For this review, take the finished solid that the model builds, in its own axes (mm). A direction names the side the tool comes from. Coordinates: 2 decimals unless noted, no trailing zeros. Loops run counter-clockwise (first coordinate to the right, second up) from the corner with the lowest first, then second, coordinate; pieces in that order, holes last. Notation, with made-up numbers: (-35, 19.25) - (15, 19.25) arc R30 ccw to (15, 57.25) - close; hole circle Ø3 at (60.25, 55). An arc over 180 degrees is marked (long way). Answer as a JSON object with one key per item and string values. Group by question number.
Item 1: Clearance check with flat-ended pins moving along their axes: pin 1 (12 mm diameter, centred on y = -629, z = 201, fed in from -X); pin 2 (12 mm diameter, centred on x = -1026, z = 425, fed in from +Y); pin 3 (3 mm diameter, centred on y = -53.5, z = 807.5, fed in from -X). State where each tip first meets the part, or that it passes through.
Item 2: Mouldability with a two-part tool opening along Z and no side actions: class faces 4 (the flat face through (-1026, -628, 810)), 5 (the flat face through (-1048, -628, 800)), 6 (the flat face through (-746, -609.913, 20)) as released by +Z, released by -Z, zero draft, split by the parting line, or undercut.
Item 3: We need section A-A (x = -589.5). Give the boundary of the cut face in (y, z), then the cut area to 3 significant figures.
Item 4: We need section D-D (x = -1019.5). Give the boundary of the cut face in (y, z), then the cut area to 3 significant figures.
Item 5: We need section C-C (y = -482). Give the boundary of the cut face in (x, z), then the cut area to 3 significant figures.
Item 6: We need section B-B (z = 541). Give the boundary of the cut face in (x, y).
Item 7: To check wall thickness, follow line 1 (X direction, y = -628, z = 774.5); line 2 (Y direction, x = -1016.5, z = 723.5); line 3 (Z direction, x = -1004.5, y = -212). State the ranges of each line that lie inside material, in increasing order.
Item 8: Tool access review of faces 1 (the flat face through (-1042.783, -630, 394)), 2 (the flat face through (-1002.783, -630, 415)), 3 (the flat face through (-1022, -49, 800)): name each direction out of +Z, -Z, +X, -X, +Y, -Y from which nothing blocks a thin tool from reaching the whole face with its end or side.
from build123d import *

# Parameters (mm, degrees)
F0_W     = 600
F0_H     = 600
F0_W_2   = 520
F0_H_2   = 520
F1_DEPTH = 40
F2_W     = 40
F2_H     = 40
F3_DEPTH = 800
F4_W     = 100
F4_H     = 100
F4_R     = 5
F5_DEPTH = 10


with BuildPart() as f1:
    # F0 (on Top) → F1 (new body)
    with BuildSketch(Plane.XY):
        with Locations((-742.534351, -349.912536)):
            Rectangle(F0_W, F0_H)
        with Locations((-742.534351, -349.912536)):
            Rectangle(F0_W_2, F0_H_2, mode=Mode.SUBTRACT)
    extrude(amount=F1_DEPTH)

    # F2 (on Top) → F3 (join)
    with BuildSketch(Plane.XY):
        with Locations((-462.971604, -70.520664)):
            Rectangle(F2_W, F2_H)
        with Locations((-1021.841088, -70.520664)):
            Rectangle(F2_W, F2_H)
        with Locations((-462.971604, -629.829387)):
            Rectangle(F2_W, F2_H)
        with Locations((-1022.782568, -629.829387)):
            Rectangle(F2_W, F2_H)
    extrude(amount=F3_DEPTH)

    # F4 (on face) → F5 (join)
    with BuildSketch(Plane.XY.offset(800)):
        with Locations((-1021.178722, -71.567007)):
            Rectangle(F4_W, F4_H)
        with Locations((-1055.047035, -105.544642)):
            Circle(F4_R, mode=Mode.SUBTRACT)
        with Locations((-985.77106, -105.544642)):
            Circle(F4_R, mode=Mode.SUBTRACT)
        with BuildLine():
            ThreePointArc((-1059.987431, -35.498975), (-1055.433054, -29.744166), (-1050.047035, -34.729242))
            ThreePointArc((-1050.047035, -34.729242), (-1050.061959, -35.115261), (-1050.106639, -35.498975))
            ThreePointArc((-1050.106639, -35.498975), (-1050.061959, -35.882689), (-1050.047035, -36.268707))
            ThreePointArc((-1050.047035, -36.268707), (-1055.433054, -41.253784), (-1059.987431, -35.498975))
        make_face(mode=Mode.SUBTRACT)
        with Locations((-985.77106, -36.268707)):
            Circle(F4_R, mode=Mode.SUBTRACT)
        with Locations((-465.089649, -71.444585)):
            Rectangle(F4_W, F4_H)
        with Locations((-498.957962, -105.42222)):
            Circle(F4_R, mode=Mode.SUBTRACT)
        with Locations((-429.681987, -105.42222)):
            Circle(F4_R, mode=Mode.SUBTRACT)
        with BuildLine():
            ThreePointArc((-503.898358, -35.376553), (-499.34398, -29.621744), (-493.957962, -34.606821))
            ThreePointArc((-493.957962, -34.606821), (-493.972885, -34.992839), (-494.017566, -35.376553))
            ThreePointArc((-494.017566, -35.376553), (-493.972885, -35.760268), (-493.957962, -36.146286))
            ThreePointArc((-493.957962, -36.146286), (-499.34398, -41.131363), (-503.898358, -35.376553))
        make_face(mode=Mode.SUBTRACT)
        with Locations((-429.681987, -36.146286)):
            Circle(F4_R, mode=Mode.SUBTRACT)
        with Locations((-463.392437, -630.738995)):
            Rectangle(F4_W, F4_H)
        with Locations((-497.260749, -664.71663)):
            Circle(F4_R, mode=Mode.SUBTRACT)
        with Locations((-427.984774, -664.71663)):
            Circle(F4_R, mode=Mode.SUBTRACT)
        with BuildLine():
            ThreePointArc((-502.201145, -594.670963), (-497.646768, -588.916154), (-492.260749, -593.901231))
            ThreePointArc((-492.260749, -593.901231), (-492.275673, -594.287249), (-492.320353, -594.670963))
            ThreePointArc((-492.320353, -594.670963), (-492.275673, -595.054678), (-492.260749, -595.440696))
            ThreePointArc((-492.260749, -595.440696), (-497.646768, -600.425773), (-502.201145, -594.670963))
        make_face(mode=Mode.SUBTRACT)
        with Locations((-427.984774, -595.440696)):
            Circle(F4_R, mode=Mode.SUBTRACT)
        with Locations((-1025.430679, -628.908239)):
            Rectangle(F4_W, F4_H)
        with Locations((-1059.298992, -662.885874)):
            Circle(F4_R, mode=Mode.SUBTRACT)
        with Locations((-990.023017, -662.885874)):
            Circle(F4_R, mode=Mode.SUBTRACT)
        with BuildLine():
            ThreePointArc((-1064.239388, -592.840207), (-1059.685011, -587.085398), (-1054.298992, -592.070474))
            ThreePointArc((-1054.298992, -592.070474), (-1054.313915, -592.456493), (-1054.358596, -592.840207))
            ThreePointArc((-1054.358596, -592.840207), (-1054.313915, -593.223921), (-1054.298992, -593.609939))
            ThreePointArc((-1054.298992, -593.609939), (-1059.685011, -598.595016), (-1064.239388, -592.840207))
        make_face(mode=Mode.SUBTRACT)
        with Locations((-990.023017, -593.609939)):
            Circle(F4_R, mode=Mode.SUBTRACT)
    extrude(amount=F5_DEPTH)


solid = f1.part
Check sheet entries:
{
 "1": {"pin 1": "stops at x = -1042.78", "pin 2": "stops at y = -50.52", "pin 3": "stops at x = -1071.18"},
 "2": {"face 4": "released by +Z", "face 5": "undercut", "face 6": "zero draft"},
 "3": {"outline": "(-649.91, 0) - (-609.91, 0) - (-609.91, 40) - (-649.91, 40) - close; (-89.91, 0) - (-49.91, 0) - (-49.91, 40) - (-89.91, 40) - close", "area": "3,200 mm2"},
 "4": {"outline": "(-678.91, 800) - (-649.83, 800) - (-649.83, 40) - (-649.91, 40) - (-649.91, 0) - (-49.91, 0) - (-49.91, 40) - (-50.52, 40) - (-50.52, 800) - (-21.57, 800) - (-21.57, 810) - (-121.57, 810) - (-121.57, 800) - (-90.52, 800) - (-90.52, 40) - (-609.83, 40) - (-609.83, 800) - (-578.91, 800) - (-578.91, 810) - (-678.91, 810) - close", "area": "86,800 mm2"},
 "5": {"outline": "(-1042.53, 0) - (-1002.53, 0) - (-1002.53, 40) - (-1042.53, 40) - close; (-482.53, 0) - (-442.53, 0) - (-442.53, 40) - (-482.53, 40) - close", "area": "3,200 mm2"},
 "6": {"outline": "(-1042.78, -649.83) - (-1002.78, -649.83) - (-1002.78, -609.83) - (-1042.78, -609.83) - close; (-1041.84, -90.52) - (-1001.84, -90.52) - (-1001.84, -50.52) - (-1041.84, -50.52) - close; (-482.97, -649.83) - (-442.97, -649.83) - (-442.97, -609.83) - (-482.97, -609.83) - close; (-482.97, -90.52) - (-442.97, -90.52) - (-442.97, -50.52) - (-482.97, -50.52) - close"},
 "7": {"line 1": "x = -1042.78 to -1002.78, -482.97 to -442.97", "line 2": "y = -649.83 to -609.83, -90.52 to -50.52", "line 3": "z = 0 to 40"},
 "8": {"face 1": "-Z, -X, +Y, -Y", "face 2": "-Y", "face 3": "none"}
}
